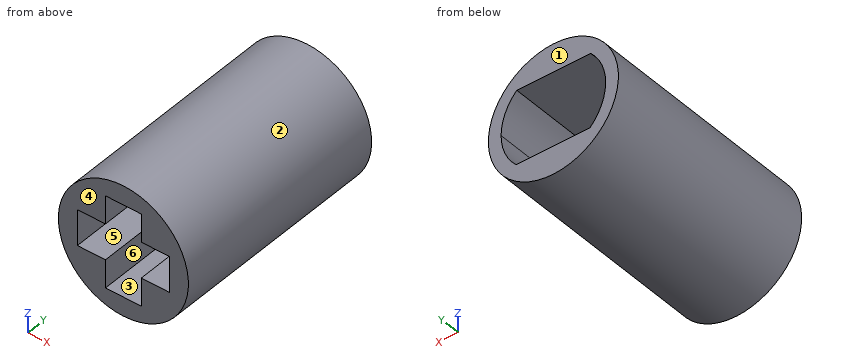
from build123d import *

# Parameters (mm, degrees)
SKETCH1_R           = 3.45
BOSS_EXTRUDE1_DEPTH = 12
CUT_EXTRUDE1_DEPTH  = 6
SKETCH3_3_W         = 1.9
SKETCH3_3_H         = 1.9
SKETCH3_3_W_2       = 1.49
SKETCH3_3_H_2       = 1.49
CUT_EXTRUDE3_DEPTH  = 6
SKETCH3_W           = 1.9
SKETCH3_H           = 1.9
SKETCH3_W_2         = 1.49
SKETCH3_H_2         = 1.49
CUT_EXTRUDE2_DEPTH  = 6


with BuildPart() as part:
    # Sketch1 → Boss-Extrude1 (new body)
    with BuildSketch(Plane(origin=(0, 0, 0), x_dir=(1, 0, 0), z_dir=(0, 1, 0))):
        with Locations(Location((0, 0, 0), (0, 0, 270))):
            Circle(SKETCH1_R)
    extrude(amount=BOSS_EXTRUDE1_DEPTH)

    # Sketch2 → Cut-Extrude1 (cut)
    with BuildSketch(Plane(origin=(0, 12, 0), x_dir=(1, 0, 0), z_dir=(0, 1, 0))):
        with BuildLine():
            Line((-1.980523516, -1.943746794), (1.943746794, -1.980523516))
            ThreePointArc((1.943746794, -1.980523516), (2.558761649, -1.073947775), (2.775, 0))
            ThreePointArc((2.775, 0), (2.568713468, 1.049921959), (1.980523516, 1.943746794))
            Line((1.980523516, 1.943746794), (-1.943746794, 1.980523516))
            ThreePointArc((-1.943746794, 1.980523516), (-2.774878148, 0.026005069), (-1.980523516, -1.943746794))
        make_face()
    extrude(amount=-CUT_EXTRUDE1_DEPTH, mode=Mode.SUBTRACT)

    # Sketch3<3> → Cut-Extrude3 (cut)
    with BuildSketch(Plane.XZ):
        Rectangle(SKETCH3_3_W, SKETCH3_3_H)
        with Locations((-1.695, 0)):
            Rectangle(SKETCH3_3_W_2, SKETCH3_3_H)
        with Locations((1.695, 0)):
            Rectangle(SKETCH3_3_W_2, SKETCH3_3_H)
        with Locations((0, -1.695)):
            Rectangle(SKETCH3_3_W, SKETCH3_3_H_2)
        with Locations((0, 1.695)):
            Rectangle(SKETCH3_3_W, SKETCH3_3_H_2)
    extrude(amount=-CUT_EXTRUDE3_DEPTH, mode=Mode.SUBTRACT)

    # Sketch3 → Cut-Extrude2 (cut)
    with BuildSketch(Plane.XZ):
        Rectangle(SKETCH3_W, SKETCH3_H)
        with Locations((-1.695, 0)):
            Rectangle(SKETCH3_W_2, SKETCH3_H)
        with Locations((0, -1.695)):
            Rectangle(SKETCH3_W, SKETCH3_H_2)
        with Locations((1.695, 0)):
            Rectangle(SKETCH3_W_2, SKETCH3_H)
        with Locations((0, 1.695)):
            Rectangle(SKETCH3_W, SKETCH3_H_2)
    extrude(amount=-CUT_EXTRUDE2_DEPTH, mode=Mode.SUBTRACT)


solid = part.part
Design review of the part built by this model. Coordinates are the model's own, in mm. Face numbers are marked on the shaded views. A direction names the side the tool comes from. Round coordinates to 2 decimals unless told otherwise and drop trailing zeros. Loops run counter-clockwise (first coordinate to the right, second up) from the corner with the lowest first, then second, coordinate; pieces in that order, holes last. Notation, with made-up numbers: (54.5, 52) - (101.5, 52) arc R37 cw to (101.5, 89) - close; hole circle Ø8 at (-17.5, -4.75). An arc over 180 degrees is marked (long way). One line per item, written item: value. Start each with the question number.
1) For the marked faces 4, 5 and 6, list the 3-axis set-ups (+Z, -Z, +X, -X, +Y, -Y) from which the entire face can be reached by the end or side of a thin tool; tool diameter is ignored.
2) Consider section A-A on y = 4. Give the boundary of the cut face in (x, z), then the cut area to 3 significant figures.
3) Consider section C-C on z = 1.5. Give the boundary of the cut face in (x, y), then the cut area to 3 significant figures.
4) Consider section B-B on x = 2.25. Give the boundary of the cut face in (y, z).
5) Insertion check: pin 1 Ø0.9 at (x, z) = (2, 1) entering from +Y; pin 2 Ø0.7 at (x, y) = (-1.5, 3) entering from +Z; pin 3 Ø1.6 at (y, z) = (3.5, -1.5) entering from -X. Each pin has a flat end and moves straight along its axis. Give the tip position at first contact, or say it passes through.
6) Draft analysis for pull direction Z (two halves, no side actions). For the marked faces 1, 2 and 3, state which applies: +Z half, -Z half, draft (parallel to the pull), parting line (faces both ways), or undercut.
7) Consider section D-D on y = 8.25. Give the boundary of the cut face in (x, z) (3 decimals), then the cut area to 3 significant figures.
8) To check wall thickness, follow L1, parallel to Y at x = -2, z = 1.25; L2, parallel to Z at x = 2.25, y = 10; L3, parallel to Z at x = 1.75, y = 10. State the ranges of each line that lie inside material, in increasing order. Write a range as from..to.
Reported:
1. face 4: +Z, -Z, +X, -X, -Y
1. face 5: +Y, -Y
1. face 6: -Y
2. outline: circle Ø6.9 at (0, 0); hole (-2.44, -0.95) - (-0.95, -0.95) - (-0.95, -2.44) - (0.95, -2.44) - (0.95, -0.95) - (2.44, -0.95) - (2.44, 0.95) - (0.95, 0.95) - (0.95, 2.44) - (-0.95, 2.44) - (-0.95, 0.95) - (-2.44, 0.95) - close
2. area: 22.5 mm^2
3. outline: (-3.11, 0) - (-0.95, 0) - (-0.95, 6) - (-2.33, 6) - (-2.33, 12) - (-3.11, 12) - close; (0.95, 0) - (3.11, 0) - (3.11, 12) - (2.33, 12) - (2.33, 6) - (0.95, 6) - close
3. area: 35.1 mm^2
4. outline: (0, -2.62) - (12, -2.62) - (12, -1.62) - (6, -1.62) - (6, -0.95) - (0, -0.95) - close; (0, 0.95) - (6, 0.95) - (6, 1.62) - (12, 1.62) - (12, 2.62) - (0, 2.62) - close
5. pin 1: stops at y = 6
5. pin 2: stops at z = 3.25
5. pin 3: stops at x = -3.38
6. face 1: draft
6. face 2: parting line
6. face 3: undercut
7. outline: circle Ø6.9 at (0, 0); hole (-1.981, 1.944) arc R2.775 ccw to (-1.944, -1.981) - (1.981, -1.944) arc R2.775 ccw to (1.944, 1.981) - close
7. area: 17.6 mm^2
8. L1: y = 0..6
8. L2: z = -2.62..-1.62, 1.62..2.62
8. L3: z = -2.97..-1.95, 1.98..2.97
